```python
from build123d import *

# Parameters (mm, degrees)
F1_DEPTH  = 150
F2_DEPTH  = 50
F3_W      = 20
F3_H      = 1250
F4_DEPTH  = 307
F5_R      = 25
F6_DEPTH  = 300.001
F7_R      = 50
F8_DEPTH  = 100
F10_DEPTH = 223
F12_DEPTH = 60
F15_R     = 40
F16_DEPTH = 320
F17_R     = 50


with BuildPart() as f1:
    # F0 (on Right) → F1 (new body, symmetric)
    with BuildSketch(Plane.YZ):
        with BuildLine():
            Line((0, 2250), (0, 0))
            Line((0, 0), (80, 0))
            Line((80, 0), (176.4553832609, 206.8492369235))
            Line((176.4553832609, 206.8492369235), (230.5361374831, 591.6537980799))
            ThreePointArc((230.5361374831, 591.6537980799), (245.1281005196, 730.4870525117), (250, 870))
            Line((250, 870), (250, 2000))
            Line((250, 2000), (0, 2250))
        make_face()
    extrude(amount=F1_DEPTH, both=True)

    # F0 (on Right) → F2 (join, symmetric)
    with BuildSketch(Plane.YZ):
        Polygon((0, 2630), (0, 2250), (250, 2000), (250, 2380), align=None)
    extrude(amount=F2_DEPTH, both=True)

    # F3 (on face) → F4 (cut)
    with BuildSketch(Plane(origin=(0, 250, 0), x_dir=(-1, 0, 0), z_dir=(0, 1, 0))):
        with Locations((0, 625)):
            Rectangle(F3_W, F3_H)
    extrude(amount=-F4_DEPTH, mode=Mode.SUBTRACT)

    # F5 (on face) → F6 (cut, through all)
    with BuildSketch(Plane(origin=(-150, 0, 0), x_dir=(0, -1, 0), z_dir=(-1, 0, 0))):
        with Locations((-80, 500)):
            Circle(F5_R)
    extrude(amount=-F6_DEPTH, mode=Mode.SUBTRACT)

    # F7 (on face) → F8 (cut, through all)
    with BuildSketch(Plane(origin=(-50, 0, 0), x_dir=(0, -1, 0), z_dir=(-1, 0, 0))):
        with Locations((-100, 2420)):
            Circle(F7_R)
    extrude(amount=-F8_DEPTH, mode=Mode.SUBTRACT)

    # F9 (on face) → F10 (cut)
    with BuildSketch(Plane.XZ):
        Polygon((150, 193.0056228459), (60, 0), (150, 0), align=None)
        Polygon((-150, 0), (-60, 0), (-150, 193.0056228459), align=None)
    extrude(amount=-F10_DEPTH, mode=Mode.SUBTRACT)

    # F11 (on Right) → F12 (cut, symmetric)
    with BuildSketch(Plane.YZ):
        with BuildLine():
            ThreePointArc((245.1281005196, 730.4870525117), (153.8671605949, 523.438334328), (189.5468692569, 300))
            Line((189.5468692569, 300), (230.5361374831, 591.6537980799))
            Line((230.5361374831, 591.6537980799), (245.1281005196, 730.4870525117))
        make_face()
        with BuildLine():
            Line((230.5361374831, 591.6537980799), (189.5468692569, 300))
            Line((189.5468692569, 300), (265.2035057545, 311.2672567368))
            Line((265.2035057545, 311.2672567368), (265.2035057545, 409.1856181622))
            Line((265.2035057545, 409.1856181622), (299.6515530456, 510.0366034563))
            Line((299.6515530456, 510.0366034563), (321.972931721, 722.4103352942))
            Line((321.972931721, 722.4103352942), (245.1281005196, 730.4870525117))
            ThreePointArc((245.1281005196, 730.4870525117), (239.0437907365, 660.9430734647), (230.5361374831, 591.6537980799))
        make_face()
        with BuildLine():
            Line((245.1281005196, 730.4870525117), (230.5361374831, 591.6537980799))
            ThreePointArc((230.5361374831, 591.6537980799), (239.0437907365, 660.9430734647), (245.1281005196, 730.4870525117))
        make_face()
    extrude(amount=F12_DEPTH, both=True, mode=Mode.SUBTRACT)

    # F15 (on face) → F16 (cut)
    with BuildSketch(Plane(origin=(0, 0, 0), x_dir=(1, 0, 0), z_dir=(0, -0.2741839815, -0.9616772558))):
        with Locations((0, -40)):
            Circle(F15_R)
    extrude(amount=-F16_DEPTH, mode=Mode.SUBTRACT)

    # F17
    f17_edges = [f1.edges().sort_by_distance(p)[0] for p in [
        (-150, 250, 1435),
        (150, 250, 1435),
        (-150, 245.128101, 730.487053),
        (-150, 203.49576, 399.251518),
        (150, 203.49576, 399.251518),
        (150, 245.128101, 730.487053),
        (-150, 0, 1221.502811),
        (150, 0, 1221.502811),
    ]]
    fillet(f17_edges, radius=F17_R)


solid = f1.part
```
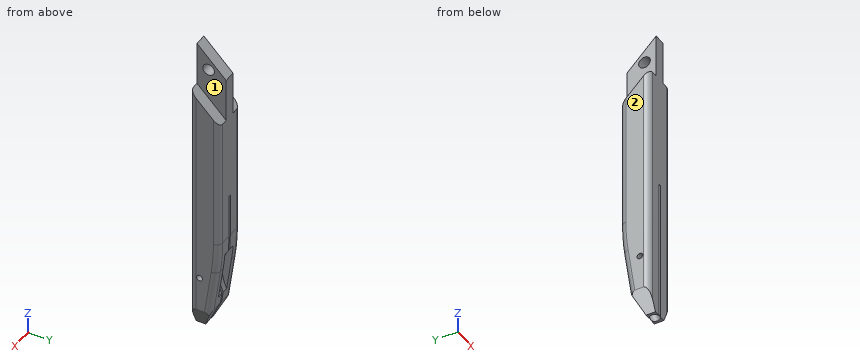
Geometry check sheet. Reference: the model listing, model coordinates, mm. Face numbers are marked on the shaded views. A direction names the side the tool comes from. Round coordinates to 2 decimals unless told otherwise and drop trailing zeros. Order: outer loops, then holes, each group sorted by start corner. A loop starts at its lowest first (then second) coordinate and runs counter-clockwise, first axis right, second up. Notation, with made-up numbers: (25, -1.5) -> (59, -1.5) arc R29 cw to (59, 21.5) -> close; hole circle Ø7 at (-7, 4.5). An arc over 180 degrees is marked (long way). Return JSON: item names as keys, results as strings. Group by question number.
Q1. Section check B-B, the plane z = 1312. Record the boundary of the cut face in (x, y).
Q2. Gauge pin test, flat ends, axial feed: pin 1 (6 mm diameter, centred on x = -1.5, y = 110.5, fed in from -Z); pin 2 (4 mm diameter, centred on x = -3, y = 97.5, fed in from +Z); pin 3 (10 mm diameter, centred on x = -50.5, y = 171.5, fed in from +Z). Record the tip position at first contact, or that the pin passes through.
Q3. Tool access check on the marked faces 1 and 2. Record the directions out of +Z, -Z, +X, -X, +Y, -Y that give a thin tool (end or side, any length) a straight path to the whole face; none if there is none.
Q4. Section check A-A, the plane z = 2420. Record the boundary of the cut face in (x, y).
Q5. Material ranges on probe 1 along Z at (x, y) = (-45, 60); probe 2 along X at (y, z) = (48.5, 668); probe 3 along X at (y, z) = (207, 1804), recorded low to high. Write a range as from..to.
Numbers:
{
 "1": {"outline": "(-150, 50) arc R50 ccw to (-100, 0) -> (100, 0) arc R50 ccw to (150, 50) -> (150, 200) arc R50 ccw to (100, 250) -> (-100, 250) arc R50 ccw to (-150, 200) -> close"},
 "2": {"pin 1": "z = 1250", "pin 2": "z = 2534.5", "pin 3": "z = 2463.47"},
 "3": {"face 1": "+Z, +X, +Y", "face 2": "+Z, -Z, -X, +Y, -Y"},
 "4": {"outline": "(-50, 0) -> (50, 0) -> (50, 50) -> (-50, 50) -> close; (-50, 150) -> (50, 150) -> (50, 210) -> (-50, 210) -> close"},
 "5": {"probe 1": "0..485, 515..2390, 2450..2570", "probe 2": "-149.98..-10, 10..149.98", "probe 3": "-149.51..149.51"}
}
